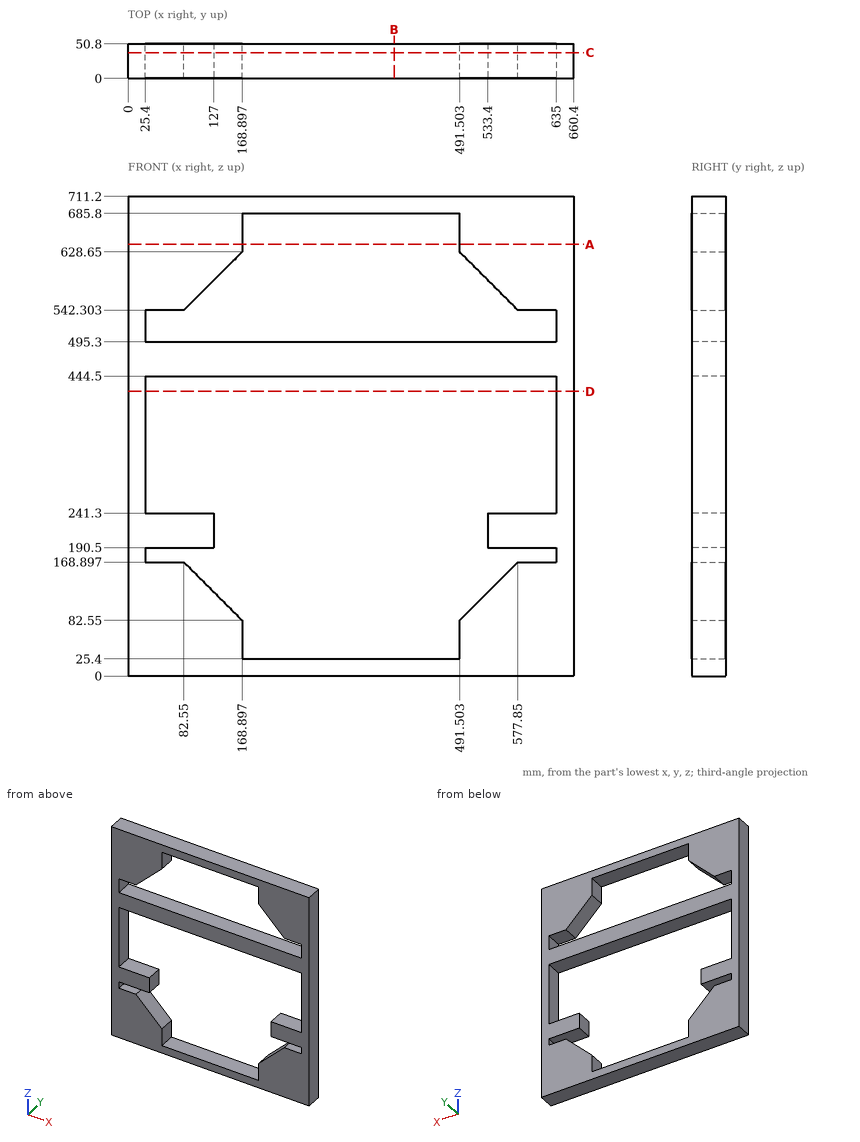
Design review of the part shown in the three views and the two pictorial views. Dimensions are in mm from the part's minimum x, y and z. Give positions to 0.01 mm unless a question says otherwise; leave off trailing zeros. Write each loop counter-clockwise with the first axis right and the second up, starting at its lowest first coordinate (ties: lowest second). Pieces come first, ordered by that corner, then holes. Notation, with made-up numbers: (73, 11) -> (108, 11) arc R20 cw to (108, 41) -> close; hole circle Ø1 at (36.25, 10.5). An arc over 180 degrees is marked (long way). Answer in a Markdown table with one row per item.
1) Add section C-C on y = 38. Count the separate pieces of the cut face and the enclosed holes in it, plus the area to 3 significant figures.
Worked answers:
| item | result |
|---|---|
| separate pieces | 1 |
| enclosed holes | 2 |
| area | 176,000 mm² |
2) Add section D-D on z = 422. State the section outline as (x, y) points.
Worked answers:
| item | result |
|---|---|
| outline | (0, 0) -> (25.4, 0) -> (25.4, 50.8) -> (0, 50.8) -> close; (635, 0) -> (660.4, 0) -> (660.4, 50.8) -> (635, 50.8) -> close |
3) Add section B-B on x = 394.5. State the section outline as (y, z) points, plus the area to 3 significant figures.
Worked answers:
| item | result |
|---|---|
| outline | (0, 0) -> (50.8, 0) -> (50.8, 25.4) -> (0, 25.4) -> close; (0, 444.5) -> (50.8, 444.5) -> (50.8, 495.3) -> (0, 495.3) -> close; (0, 685.8) -> (50.8, 685.8) -> (50.8, 711.2) -> (0, 711.2) -> close |
| area | 5,160 mm² |
4) For L1, parallel to Z at x = 623, y = 25.5; L2, parallel to Z at x = 296.5, y = 42.5; L3, parallel to X at y = 48, z = 518, list the stretches that pass through material, from the lowest coordinate up. Write a range as [from, to].
Worked answers:
| item | result |
|---|---|
| L1 | [0, 168.9], [190.5, 241.3], [444.5, 495.3], [542.3, 711.2] |
| L2 | [0, 25.4], [444.5, 495.3], [685.8, 711.2] |
| L3 | [0, 25.4], [635, 660.4] |
5) Add section A-A on z = 640. State the section outline as (x, y) points, plus the area to 3 significant figures.
Worked answers:
| item | result |
|---|---|
| outline | (0, 0) -> (168.9, 0) -> (168.9, 50.8) -> (0, 50.8) -> close; (491.5, 0) -> (660.4, 0) -> (660.4, 50.8) -> (491.5, 50.8) -> close |
| area | 17,200 mm² |
